Check sheet for the modelled part. Datum: model origin and axes. Units: mm. Face numbers are marked on the shaded views. A direction names the side the tool comes from. Round coordinates to 2 decimals unless told otherwise and drop trailing zeros. Order: outer loops, then holes, each group sorted by start corner. A loop starts at its lowest first (then second) coordinate and runs counter-clockwise, first axis right, second up.
```python
from build123d import *

# Parameters (mm, degrees)
SKETCH1_W           = 76.5
SKETCH1_H           = 45
SKETCH1_R           = 1.25
BOSS_EXTRUDE1_DEPTH = 5
SKETCH2_W           = 9
SKETCH2_H           = 9
SKETCH2_R           = 2.25
BOSS_EXTRUDE2_DEPTH = 25
CHAMFER1_SIZE       = 1
CHAMFER2_SIZE       = 3


with BuildPart() as part:
    # Sketch1 → Boss-Extrude1 (new body)
    with BuildSketch(Plane(origin=(0, 0, 0), x_dir=(1, 0, 0), z_dir=(0, 1, 0))):
        with Locations((38.25, 22.5)):
            Rectangle(SKETCH1_W, SKETCH1_H)
        with Locations(Location((9.75, 32.75, 0), (0, 0, 270))):
            Circle(SKETCH1_R, mode=Mode.SUBTRACT)
        with Locations(Location((9.75, 12.25, 0), (0, 0, 270))):
            Circle(SKETCH1_R, mode=Mode.SUBTRACT)
        with Locations(Location((66.75, 12.25, 0), (0, 0, 270))):
            Circle(SKETCH1_R, mode=Mode.SUBTRACT)
        with Locations(Location((66.75, 32.75, 0), (0, 0, 270))):
            Circle(SKETCH1_R, mode=Mode.SUBTRACT)
        with BuildLine():
            Line((13.75, 34.080542855), (62.75, 34.080542855))
            ThreePointArc((62.75, 34.080542855), (64.080542855, 32.75), (62.75, 31.419457145))
            Line((62.75, 31.419457145), (13.75, 31.419457145))
            ThreePointArc((13.75, 31.419457145), (12.419457145, 32.75), (13.75, 34.080542855))
        make_face(mode=Mode.SUBTRACT)
        with BuildLine():
            Line((13.75, 13.352251527), (62.75, 13.352251527))
            ThreePointArc((62.75, 13.352251527), (63.852251527, 12.25), (62.75, 11.147748473))
            Line((62.75, 11.147748473), (13.75, 11.147748473))
            ThreePointArc((13.75, 11.147748473), (12.647748473, 12.25), (13.75, 13.352251527))
        make_face(mode=Mode.SUBTRACT)
    extrude(amount=BOSS_EXTRUDE1_DEPTH)

    # Sketch2 → Boss-Extrude2 (add)
    # profile 1 of 4: a face of its own
    with BuildSketch(Plane(origin=(0, 5, 0), x_dir=(1, 0, 0), z_dir=(0, 1, 0))):
        with Locations((4.5, 40.5)):
            Rectangle(SKETCH2_W, SKETCH2_H)
        with Locations(Location((4.5, 40.5, 0), (0, 0, 270))):
            Circle(SKETCH2_R, mode=Mode.SUBTRACT)
    # profile 2 of 4: a face of its own
    with BuildSketch(Plane(origin=(0, 5, 0), x_dir=(1, 0, 0), z_dir=(0, 1, 0))):
        with Locations((4.5, 4.5)):
            Rectangle(SKETCH2_W, SKETCH2_H)
        with Locations(Location((4.5, 4.5, 0), (0, 0, 270))):
            Circle(SKETCH2_R, mode=Mode.SUBTRACT)
    # profile 3 of 4: a face of its own
    with BuildSketch(Plane(origin=(0, 5, 0), x_dir=(1, 0, 0), z_dir=(0, 1, 0))):
        with Locations((72, 4.5)):
            Rectangle(SKETCH2_W, SKETCH2_H)
        with Locations(Location((72, 4.5, 0), (0, 0, 270))):
            Circle(SKETCH2_R, mode=Mode.SUBTRACT)
    # profile 4 of 4: a face of its own
    with BuildSketch(Plane(origin=(0, 5, 0), x_dir=(1, 0, 0), z_dir=(0, 1, 0))):
        with Locations((72, 40.5)):
            Rectangle(SKETCH2_W, SKETCH2_H)
        with Locations(Location((72, 40.5, 0), (0, 0, 270))):
            Circle(SKETCH2_R, mode=Mode.SUBTRACT)
    extrude(amount=BOSS_EXTRUDE2_DEPTH)

    # Chamfer1
    chamfer1_edges = [part.edges().sort_by_distance(p)[0] for p in [
        (76.5, 30, -40.5),
        (72, 30, -45),
        (67.5, 30, -40.5),
        (72, 30, -36),
        (0, 30, -40.5),
        (4.5, 30, -36),
        (9, 30, -40.5),
        (4.5, 30, -45),
        (0, 30, -4.5),
        (4.5, 30, 0),
        (9, 30, -4.5),
        (4.5, 30, -9),
        (0, 15, -45),
        (76.5, 15, -45),
        (76.5, 15, 0),
        (0, 15, 0),
        (76.5, 30, -4.5),
        (72, 30, -9),
        (67.5, 30, -4.5),
        (72, 30, 0),
    ]]
    chamfer(chamfer1_edges, length=CHAMFER1_SIZE)

    # Chamfer2
    # the kernel refuses this chamfer: 3 mm, written as the material it adds along each edge
    with BuildSketch(Plane(origin=(67.5, 5, -45), x_dir=(-1, 0, 0), z_dir=(0, 0, 1))) as chamfer2_piece_1_section:
        Polygon((CHAMFER2_SIZE, 0), (0, -CHAMFER2_SIZE), (0, 0), align=None)
    chamfer2_piece_1 = extrude(amount=16.715048964, mode=Mode.PRIVATE)
    chamfer2_piece_1 = chamfer2_piece_1 - Plane(origin=(66.75, 5, -32.75), x_dir=(0, 0, 1), z_dir=(0, -1, 0)) * Cylinder(1.25, 46, mode=Mode.PRIVATE)
    chamfer2_piece_1 = split(chamfer2_piece_1, bisect_by=Plane(origin=(67.5, 11, -39), z_dir=(0, -0.7071067811865476, -0.7071067811865476)), keep=Keep.TOP, mode=Mode.PRIVATE)
    add(chamfer2_piece_1)
    with BuildSketch(Plane(origin=(59.784951036, 5, -36), x_dir=(0, 0, 1), z_dir=(1, 0, 0))) as chamfer2_piece_2_section:
        Polygon((CHAMFER2_SIZE, 0), (0, -CHAMFER2_SIZE), (0, 0), align=None)
    chamfer2_piece_2 = extrude(amount=16.715048964, mode=Mode.PRIVATE)
    chamfer2_piece_2 = chamfer2_piece_2 - Plane(origin=(66.75, 5, -32.75), x_dir=(0, 0, 1), z_dir=(0, -1, 0)) * Cylinder(1.25, 46, mode=Mode.PRIVATE)
    chamfer2_piece_2 = split(chamfer2_piece_2, bisect_by=Plane(origin=(62.142475518, 2.642475518, -36), z_dir=(0.7071067811865476, -0.7071067811865476, 1.1165101928417953e-15)), keep=Keep.TOP, mode=Mode.PRIVATE)
    add(chamfer2_piece_2)
    with BuildSketch(Plane(origin=(16.715048964, 5, -36), x_dir=(0, 0, 1), z_dir=(-1, 0, 0))) as chamfer2_piece_3_section:
        Polygon((CHAMFER2_SIZE, 0), (0, CHAMFER2_SIZE), (0, 0), align=None)
    chamfer2_piece_3 = extrude(amount=16.715048964, mode=Mode.PRIVATE)
    chamfer2_piece_3 = chamfer2_piece_3 - Plane(origin=(9.75, 5, -32.75), x_dir=(0, 0, 1), z_dir=(0, -1, 0)) * Cylinder(1.25, 46, mode=Mode.PRIVATE)
    chamfer2_piece_3 = split(chamfer2_piece_3, bisect_by=Plane(origin=(14.357524482, 2.642475518, -36), z_dir=(-0.7071067811865476, -0.7071067811865476, 0)), keep=Keep.TOP, mode=Mode.PRIVATE)
    add(chamfer2_piece_3)
    with BuildSketch(Plane(origin=(9, 5, -45), x_dir=(1, 0, 0), z_dir=(0, 0, 1))) as chamfer2_piece_4_section:
        Polygon((CHAMFER2_SIZE, 0), (0, CHAMFER2_SIZE), (0, 0), align=None)
    chamfer2_piece_4 = extrude(amount=16.715048964, mode=Mode.PRIVATE)
    chamfer2_piece_4 = chamfer2_piece_4 - Plane(origin=(9.75, 5, -32.75), x_dir=(0, 0, 1), z_dir=(0, -1, 0)) * Cylinder(1.25, 46, mode=Mode.PRIVATE)
    chamfer2_piece_4 = split(chamfer2_piece_4, bisect_by=Plane(origin=(9, 11, -39), z_dir=(0, -0.7071067811865476, -0.7071067811865476)), keep=Keep.TOP, mode=Mode.PRIVATE)
    add(chamfer2_piece_4)
    with BuildSketch(Plane(origin=(9, 5, 0), x_dir=(0, 1, 0), z_dir=(0, 0, -1))) as chamfer2_piece_5_section:
        Polygon((CHAMFER2_SIZE, 0), (0, CHAMFER2_SIZE), (0, 0), align=None)
    chamfer2_piece_5 = extrude(amount=16.715048964, mode=Mode.PRIVATE)
    chamfer2_piece_5 = chamfer2_piece_5 - Plane(origin=(9.75, 5, -12.25), x_dir=(0, 0, 1), z_dir=(0, -1, 0)) * Cylinder(1.25, 46, mode=Mode.PRIVATE)
    chamfer2_piece_5 = split(chamfer2_piece_5, bisect_by=Plane(origin=(9, 11, -6), z_dir=(0, -0.7071067811865476, 0.7071067811865476)), keep=Keep.TOP, mode=Mode.PRIVATE)
    add(chamfer2_piece_5)
    with BuildSketch(Plane(origin=(16.715048964, 5, -9), x_dir=(0, 0, -1), z_dir=(-1, 0, 0))) as chamfer2_piece_6_section:
        Polygon((CHAMFER2_SIZE, 0), (0, -CHAMFER2_SIZE), (0, 0), align=None)
    chamfer2_piece_6 = extrude(amount=16.715048964, mode=Mode.PRIVATE)
    chamfer2_piece_6 = chamfer2_piece_6 - Plane(origin=(9.75, 5, -12.25), x_dir=(0, 0, 1), z_dir=(0, -1, 0)) * Cylinder(1.25, 46, mode=Mode.PRIVATE)
    chamfer2_piece_6 = split(chamfer2_piece_6, bisect_by=Plane(origin=(14.357524482, 2.642475518, -9), z_dir=(-0.7071067811865474, -0.7071067811865478, 0)), keep=Keep.TOP, mode=Mode.PRIVATE)
    add(chamfer2_piece_6)
    with BuildSketch(Plane(origin=(59.784951036, 5, -9), x_dir=(0, 0, -1), z_dir=(1, 0, 0))) as chamfer2_piece_7_section:
        Polygon((CHAMFER2_SIZE, 0), (0, CHAMFER2_SIZE), (0, 0), align=None)
    chamfer2_piece_7 = extrude(amount=16.715048964, mode=Mode.PRIVATE)
    chamfer2_piece_7 = chamfer2_piece_7 - Plane(origin=(66.75, 5, -12.25), x_dir=(0, 0, 1), z_dir=(0, -1, 0)) * Cylinder(1.25, 46, mode=Mode.PRIVATE)
    chamfer2_piece_7 = split(chamfer2_piece_7, bisect_by=Plane(origin=(62.142475518, 2.642475518, -9), z_dir=(0.7071067811865476, -0.7071067811865476, 0)), keep=Keep.TOP, mode=Mode.PRIVATE)
    add(chamfer2_piece_7)
    with BuildSketch(Plane(origin=(67.5, 5, 0), x_dir=(-1, 0, 0), z_dir=(0, 0, -1))) as chamfer2_piece_8_section:
        Polygon((CHAMFER2_SIZE, 0), (0, CHAMFER2_SIZE), (0, 0), align=None)
    chamfer2_piece_8 = extrude(amount=16.715048964, mode=Mode.PRIVATE)
    chamfer2_piece_8 = chamfer2_piece_8 - Plane(origin=(66.75, 5, -12.25), x_dir=(0, 0, 1), z_dir=(0, -1, 0)) * Cylinder(1.25, 46, mode=Mode.PRIVATE)
    chamfer2_piece_8 = split(chamfer2_piece_8, bisect_by=Plane(origin=(67.5, 11, -6), z_dir=(0, -0.7071067811865476, 0.7071067811865476)), keep=Keep.TOP, mode=Mode.PRIVATE)
    add(chamfer2_piece_8)


solid = part.part
```
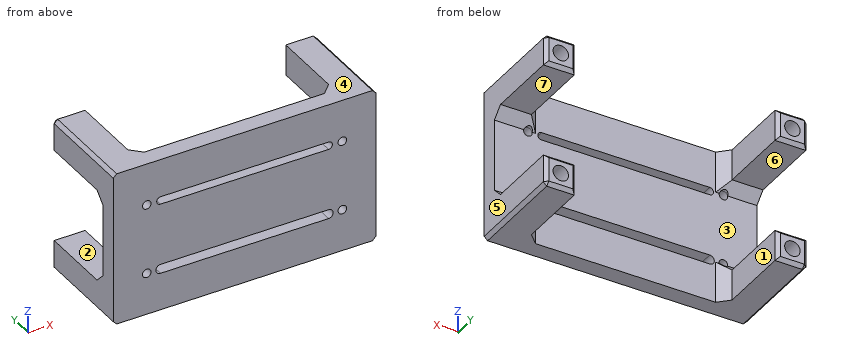
Item 1: Go/stop test with flat-tipped pins: P1, Ø1.5, axis at x = 62.5, z = -8, coming from the +Y side; P2, Ø3, axis at x = 66.75, z = -12.25, coming from the +Y side; P3, Ø2, axis at x = 9.75, z = -12.25, coming from the -Y side. Record where each tip stops, or that it passes through.
Answer:
P1: stops at y = 5
P2: stops at y = 6.25
P3: passes through
Item 2: Sectioned sample at D-D (z = -10). Record the cut outline in (x, y), and give its area (4 significant figures).
Answer:
outline: (0, 0) - (76.5, 0) - (76.5, 7) - (66.5, 7) - (64.5, 5) - (12, 5) - (10, 7) - (0, 7) - close
area: 426.5 mm2
Item 3: Sectioned sample at B-B (x = 66.75). Record the cut outline in (y, z), and give its area (3 significant figures).
Answer:
outline: (0, -45) - (7.25, -45) - (7.25, -35.25) - (6, -34) - (0, -34) - close; (0, -31.5) - (5, -31.5) - (5, -13.5) - (0, -13.5) - close; (0, -11) - (6, -11) - (7.25, -9.75) - (7.25, 0) - (0, 0) - close
area: 248 mm2
Item 4: Sectioned sample at A-A (y = 15.75). Record the cut outline in (x, z).
Answer:
outline: (0, -44) - (1, -45) - (9, -45) - (9, -36) - (0, -36) - close; (0, -9) - (9, -9) - (9, 0) - (1, 0) - (0, -1) - close; (67.5, -45) - (75.5, -45) - (76.5, -44) - (76.5, -36) - (67.5, -36) - close; (67.5, -9) - (76.5, -9) - (76.5, -1) - (75.5, 0) - (67.5, 0) - close; hole circle Ø4.5 at (4.5, -40.5); hole circle Ø4.5 at (4.5, -4.5); hole circle Ø4.5 at (72, -40.5); hole circle Ø4.5 at (72, -4.5)
Item 5: Scan lines: line 1 along X through (y, z) = (22.5, -40.5); line 2 along Z through (x, y) = (9.75, 1.15); line 3 along Z through (x, y) = (28, 3.75). Record each from-to range of solid material in increasing order.
Answer:
line 1: x = 0 to 2.25, 6.75 to 9, 67.5 to 69.75, 74.25 to 76.5
line 2: z = -45 to -34, -31.5 to -13.5, -11 to 0
line 3: z = -45 to -34.08, -31.42 to -13.35, -11.15 to 0
Item 6: Access from +Z, -Z, +X, -X, +Y, -Y to the whole of each face (thin tool, end or side, straight path). Record for the marked faces 1, 2 and 3.
Answer:
face 1: +Z, -Z, +Y
face 2: +X, -X, +Y
face 3: +Y
Item 7: Sectioned sample at C-C (z = -4.5). Record the cut outline in (x, y).
Answer:
outline: (0, 0) - (76.5, 0) - (76.5, 29) - (75.5, 30) - (74.25, 30) - (74.25, 5) - (69.75, 5) - (69.75, 30) - (68.5, 30) - (67.5, 29) - (67.5, 8) - (64.5, 5) - (12, 5) - (9, 8) - (9, 29) - (8, 30) - (6.75, 30) - (6.75, 5) - (2.25, 5) - (2.25, 30) - (1, 30) - (0, 29) - close
Item 8: Release check for a two-part mould opening along Z. For the marked faces 4, 5, 6 and 7 record: released by +Z, released by -Z, zero draft, split by the parting line, or undercut.
Answer:
face 4: released by +Z
face 5: zero draft
face 6: undercut
face 7: undercut
